```python
from build123d import *

# Parameters (mm, degrees)
SKETCH1_W           = 37
SKETCH1_H           = 10
BOSS_EXTRUDE1_DEPTH = 2
SKETCH2_W           = 16
SKETCH2_H           = 10
BOSS_EXTRUDE2_DEPTH = 10.5
SKETCH3_R           = 2.75
CUT_EXTRUDE1_DEPTH  = 41.314389491
SKETCH4_R           = 2.25
CUT_EXTRUDE2_DEPTH  = 10
CHAMFER1_SIZE       = 3


with BuildPart() as part:
    # Sketch1 → Boss-Extrude1 (new body)
    with BuildSketch(Plane(origin=(0, 0, 0), x_dir=(1, 0, 0), z_dir=(0, 1, 0))):
        with Locations((18.5, 5)):
            Rectangle(SKETCH1_W, SKETCH1_H)
    extrude(amount=BOSS_EXTRUDE1_DEPTH)

    # Sketch2 → Boss-Extrude2 (add)
    with BuildSketch(Plane(origin=(0, 2, 0), x_dir=(1, 0, 0), z_dir=(0, 1, 0))):
        with Locations((18.5, 5)):
            Rectangle(SKETCH2_W, SKETCH2_H)
    extrude(amount=BOSS_EXTRUDE2_DEPTH)

    # Sketch3 → Cut-Extrude1 (cut, through all)
    with BuildSketch(Plane(origin=(0, 0, -10), x_dir=(-1, 0, 0), z_dir=(0, 0, -1))):
        with Locations((-18.5, 6.25)):
            Circle(SKETCH3_R)
    extrude(amount=-CUT_EXTRUDE1_DEPTH, mode=Mode.SUBTRACT)

    # Sketch4 → Cut-Extrude2 (cut)
    with BuildSketch(Plane(origin=(0, 2, 0), x_dir=(1, 0, 0), z_dir=(0, 1, 0))):
        with Locations(Location((5.25, 5, 0), (0, 0, 270))):
            Circle(SKETCH4_R)
        with Locations(Location((31.75, 5, 0), (0, 0, 270))):
            Circle(SKETCH4_R)
    extrude(amount=-CUT_EXTRUDE2_DEPTH, mode=Mode.SUBTRACT)

    # Chamfer1
    chamfer1_edges = [part.edges().sort_by_distance(p)[0] for p in [
        (0, 1, -10),
        (37, 1, -10),
        (37, 1, 0),
        (0, 1, 0),
    ]]
    chamfer(chamfer1_edges, length=CHAMFER1_SIZE)


solid = part.part
```
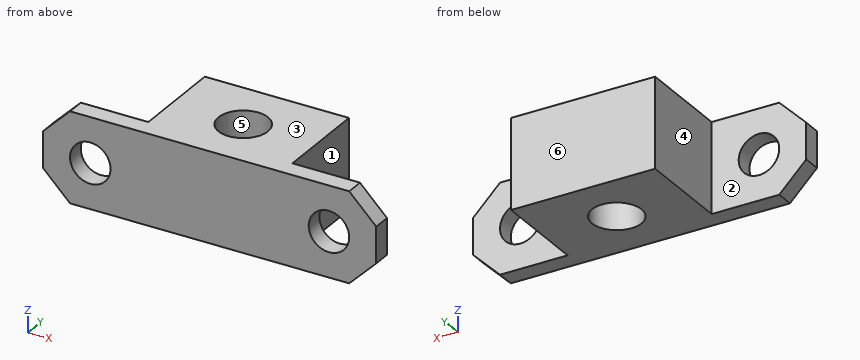
Can you work these out from the model? Positions are in its coordinate system, mm. Face numbers are marked on the shaded views. A direction names the side the tool comes from. Coordinates: 2 decimals unless noted, no trailing zeros. Loops run counter-clockwise (first coordinate to the right, second up) from the corner with the lowest first, then second, coordinate; pieces in that order, holes last.
Item 1: Suppose I cut it at A-A (z = -5). Please give me the cut outline in (x, y).
Answers below:
outline: (0, 0) - (3, 0) - (3, 2) - (0, 2) - close; (7.5, 0) - (29.5, 0) - (29.5, 2) - (26.5, 2) - (26.5, 12.5) - (10.5, 12.5) - (10.5, 2) - (7.5, 2) - close; (34, 0) - (37, 0) - (37, 2) - (34, 2) - close; hole circle Ø5.5 at (18.5, 6.25)
Item 2: Suppose I cut it at B-B (x = 18.5). Please give me the cut outline in (y, z), then the cut area to 3 significant figures.
Answers below:
outline: (0, -10) - (3.5, -10) - (3.5, 0) - (0, 0) - close; (9, -10) - (12.5, -10) - (12.5, 0) - (9, 0) - close
area: 70.0 mm2
Item 3: If we mould it in two halves opening along X, with no side actions, what happens to the marked faces 4, 5 and 6? For each: released by +X, released by -X, zero draft, split by the parting line, or undercut.
Answers below:
face 4: released by -X
face 5: undercut
face 6: zero draft
Item 4: I'm going to push flat-ended pins straight in: pin 1 (6 mm diameter, centred on x = 31.75, z = -5, fed in from +Y); pin 2 (3 mm diameter, centred on y = 9.5, z = -6.5, fed in from +X). Where does each tip first touch, or does it pass through?
Answers below:
pin 1: stops at y = 2
pin 2: stops at x = 26.5
Item 5: Suppose I cut it at D-D (z = -2). Please give me the cut outline in (x, y), then the cut area to 3 significant figures.
Answers below:
outline: (1, 0) - (36, 0) - (36, 2) - (26.5, 2) - (26.5, 12.5) - (10.5, 12.5) - (10.5, 2) - (1, 2) - close; hole circle Ø5.5 at (18.5, 6.25)
area: 214 mm2
Item 6: Please list where these lines run through material, in increasing order: L1, parallel to X at y = 9.25, z = -2; L2, parallel to X at y = 7, z = -7.5; L3, parallel to Y at x = 18, z = -8.
Answers below:
L1: x = 10.5 to 26.5
L2: x = 10.5 to 15.85, 21.15 to 26.5
L3: y = 0 to 3.55, 8.95 to 12.5
Item 7: Which directions (+Z, -Z, +X, -X, +Y, -Y) give clear straight access to the entire face, cutting with the end or side of a thin tool? Please do the marked faces 1, 2 and 3.
Answers below:
face 1: +Z, -Z, +X, +Y
face 2: +Z, -Z, -X, +Y
face 3: +Z, +X, -X, +Y, -Y
Item 8: Suppose I cut it at C-C (y = 4). Please give me the cut outline in (x, z), then the cut area to 3 significant figures.
Answers below:
outline: (10.5, -10) - (16.92, -10) - (16.92, 0) - (10.5, 0) - close; (20.08, -10) - (26.5, -10) - (26.5, 0) - (20.08, 0) - close
area: 128 mm2
